Read the model definition and answer for the solid it produces. Units are mm, in the model's axes. Give positions to 0.01 mm unless a question says otherwise; leave off trailing zeros. Order: outer loops, then holes, each group sorted by start corner. A loop starts at its lowest first (then second) coordinate and runs counter-clockwise, first axis right, second up.
Item 1: A cutting plane is placed at C-C (z = -35). Write down the section's boundary in (x, y).
Item 2: A cutting plane is placed at B-B (x = 132.5). Write down the section's boundary in (y, z), plus the area to 3 significant figures.
Item 3: A cutting plane is placed at A-A (z = -62.5). Write down the section's boundary in (x, y).
Item 4: A cutting plane is placed at D-D (y = 2.05). State how many separate pieces and enclosed holes the cut face has, plus the area to 3 significant figures.
Item 5: Find the intervals of material crossed by line 1 along X through (y, z) = (2.15, -35); line 2 along X through (y, z) = (2.15, -7.5); line 3 along Z through (x, y) = (24, 2.35), in increasing order.
Item 6: Given pin 1 Ø12 at (x, z) = (62, -37) entering from -Y, flat-ended and moving along its own axis, determine where the tip first touches the part or whether it passes through.
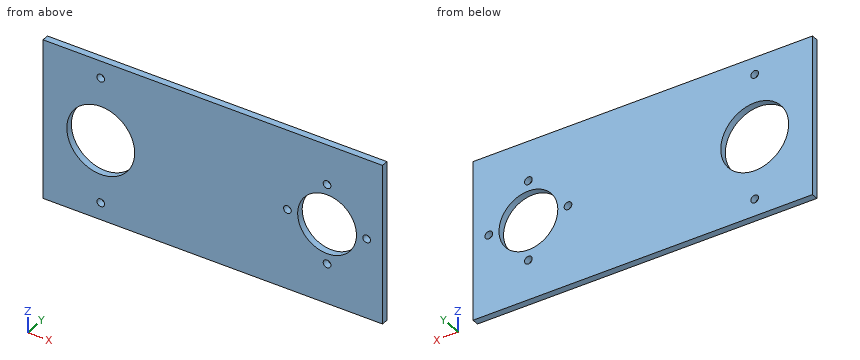
from build123d import *

# Parameters (mm, degrees)
SKETCH1_W            = 150
SKETCH1_H            = 70
BOSS_EXTRUDE1_DEPTH  = 3
SKETCH2_R            = 15
SKETCH2_R_2          = 13
CUT_EXTRUDE1_DEPTH   = 166.556636835
M3_CLEARANCE_HOLE1_D = 3.4


with BuildPart() as part:
    # Sketch1 → Boss-Extrude1 (new body)
    with BuildSketch(Plane(origin=(0, 0, 0), x_dir=(1, 0, 0), z_dir=(0, 1, 0))):
        with Locations((75, 35)):
            Rectangle(SKETCH1_W, SKETCH1_H)
    extrude(amount=BOSS_EXTRUDE1_DEPTH)

    # Sketch2 → Cut-Extrude1 (cut, through all)
    with BuildSketch(Plane(origin=(0, 3, 0), x_dir=(1, 0, 0), z_dir=(0, 1, 0))):
        with Locations(Location((25.522198067, 35, 0), (0, 0, 270))):
            Circle(SKETCH2_R)
        with Locations(Location((125.522198067, 35, 0), (0, 0, 270))):
            Circle(SKETCH2_R_2)
    extrude(amount=-CUT_EXTRUDE1_DEPTH, mode=Mode.SUBTRACT)

    # M3 Clearance Hole1 (through all)
    with Locations(Plane(origin=(0, 3, 0), x_dir=(1, 0, 0), z_dir=(0, 1, 0))):
        with Locations((25.522198067, 62.5), (25.522198067, 7.5), (108.022198067, 35), (125.522198067, 52.5), (143.022198067, 35), (125.522198067, 17.5)):
            Hole(M3_CLEARANCE_HOLE1_D / 2)


solid = part.part
Response values:
1. outline: (0, 0) - (10.52, 0) - (10.52, 3) - (0, 3) - close; (40.52, 0) - (106.32, 0) - (106.32, 3) - (40.52, 3) - close; (109.72, 0) - (112.52, 0) - (112.52, 3) - (109.72, 3) - close; (138.52, 0) - (141.32, 0) - (141.32, 3) - (138.52, 3) - close; (144.72, 0) - (150, 0) - (150, 3) - (144.72, 3) - close
2. outline: (0, -70) - (3, -70) - (3, -45.97) - (0, -45.97) - close; (0, -24.03) - (3, -24.03) - (3, 0) - (0, 0) - close
2. area: 144 mm2
3. outline: (0, 0) - (23.82, 0) - (23.82, 3) - (0, 3) - close; (27.22, 0) - (150, 0) - (150, 3) - (27.22, 3) - close
4. separate pieces: 1
4. enclosed holes: 8
4. area: 9,210 mm2
5. line 1: x = 0 to 10.52, 40.52 to 106.32, 109.72 to 112.52, 138.52 to 141.32, 144.72 to 150
5. line 2: x = 0 to 23.82, 27.22 to 150
5. line 3: z = -70 to -63.26, -61.74 to -49.92, -20.08 to -8.26, -6.74 to 0
6. pin 1: stops at y = 0
